from build123d import *

# Parameters (mm, degrees)
BODYSKE_R      = 33.5
BODYSKE_R_2    = 25.25
BASEBODY_DEPTH = 8
SLIT_DEPTH     = 49.046852134
FILLET1_R      = 2


with BuildPart() as part:
    # BodySke → BaseBody (new body)
    with BuildSketch(Plane(origin=(0, 0, 0), x_dir=(1, 0, 0), z_dir=(0, 1, 0))):
        with Locations(Location((0, 0, 0), (0, 0, 270))):
            Circle(BODYSKE_R)
        with Locations(Location((0, 0, 0), (0, 0, 270))):
            Circle(BODYSKE_R_2, mode=Mode.SUBTRACT)
    extrude(amount=BASEBODY_DEPTH)

    # SlitSke → Slit (cut, through all)
    with BuildSketch(Plane.XY):
        Polygon((0, 0), (-4.618802154, 8), (0, 8), (4.618802154, 0), align=None)
    extrude(amount=SLIT_DEPTH, mode=Mode.SUBTRACT)

    # Fillet1
    fillet1_edges = [part.edges().sort_by_distance(p)[0] for p in [
        (-2.319204626, 0, -25.143265299),
        (2.319204626, 8, -25.143265299),
    ]]
    fillet(fillet1_edges, radius=FILLET1_R)


solid = part.part
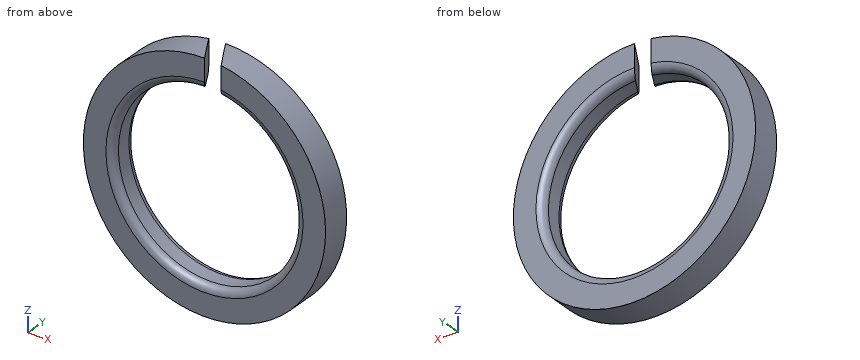
Part model, mm, in its own coordinate system. Coordinates: 2 decimals unless noted, no trailing zeros. Loops run counter-clockwise (first coordinate to the right, second up) from the corner with the lowest first, then second, coordinate; pieces in that order, holes last. Notation, with made-up numbers: M 5.25,-36 L 57.25,-36 A23 ccw 57.25,-15 Z; hole C -19,80 d1. An arc over 180 degrees is marked long. Use a Markdown table: item, result. Add a question column.
Q1. Probe L1, parallel to X at y = 4.35, z = 0; L2, parallel to X at y = 6.25, z = -0.5; L3, parallel to Z at x = 0, y = 4.6. List the from-to ranges inside material, lowest first.
Q2. Cut at A-A (z = 0). Write the cut outline in (x, y).
Q3. Pin check, flat tips, straight feed: P1, Ø2, axis at y = 3.5, z = -25.5, coming from the +X side; P2, Ø4, axis at x = 8, y = 1, coming from the -Z side; P3, Ø2, axis at x = 11, y = 4, coming from the +Z side. Stop position of each tip, or through.
Q4. Cut at B-B (y = 3). Write the cut outline in (x, z).
Worked out:
| question | item | result |
|---|---|---|
| 1 | L1 | x = -33.5 to -25.25, 25.25 to 33.5 |
| 1 | L2 | x = -33.5 to -25.26, 25.26 to 33.5 |
| 1 | L3 | z = -33.5 to -25.25 |
| 2 | outline | M -33.5,0 L -27.25,0 A2 ccw -25.25,2 L -25.25,6 A2 ccw -27.25,8 L -33.5,8 Z; M 25.25,2 A2 ccw 27.25,0 L 33.5,0 L 33.5,8 L 27.25,8 A2 ccw 25.25,6 Z |
| 3 | P1 | stops at x = 22.85 |
| 3 | P2 | stops at z = -32.96 |
| 3 | P3 | stops at z = 31.97 |
| 4 | outline | M -1.73,25.19 L -1.73,33.46 A33.5 ccw long 2.89,33.38 L 2.89,25.08 A25.25 cw long Z |
